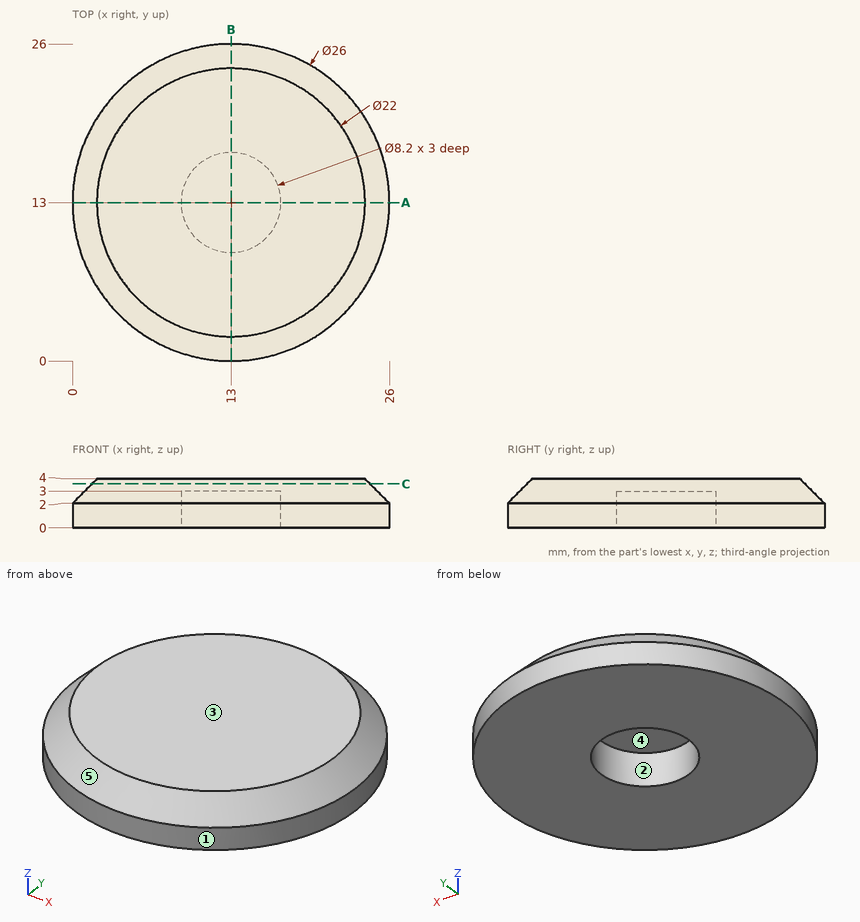
Input: dimensioned drawing with shaded views. Units: mm. Origin: part minimum x, y, z. A direction names the side the tool comes from. Give positions to 0.01 mm unless a question says otherwise; leave off trailing zeros. Order: outer loops, then holes, each group sorted by start corner. A loop starts at its lowest first (then second) coordinate and runs counter-clockwise, first axis right, second up.
(1) Access query for the marked faces 1 and 2. Directions: +Z, -Z, +X, -X, +Y, -Y. A direction counts if a zero-diameter tool reaches every point of the face in a straight line with its end or side. Return the directions, or none.
(2) Section query C-C (z = 3.6). Return the cut outline in (x, y), plus the area to 3 significant figures.
(3) Material intervals for line 1 along Y through (x, z) = (13, 1); line 2 along Y through (x, z) = (13, 2.35); line 3 along Z through (x, y) = (13.5, 16.5), sorted ascending.
(4) Section query A-A (y = 13). Return the cut outline in (x, z).
(5) Pull-direction query (Y, two-part tool) for the marked faces 3, 4 and 5; classes: +Y half, -Y half, draft (parallel to the pull), parting line (faces both ways), or undercut.
Outcome:
1. face 1: +Z, -Z
1. face 2: -Z
2. outline: circle Ø22.8 at (13, 13)
2. area: 408 mm2
3. line 1: y = 0 to 8.9, 17.1 to 26
3. line 2: y = 0.35 to 8.9, 17.1 to 25.65
3. line 3: z = 3 to 4
4. outline: (0, 0) - (8.9, 0) - (8.9, 3) - (17.1, 3) - (17.1, 0) - (26, 0) - (26, 2) - (24, 4) - (2, 4) - (0, 2) - close
5. face 3: draft
5. face 4: undercut
5. face 5: parting line
